from build123d import *

# Parameters (mm, degrees)
SKETCH1_R                = 50
BOSS_EXTRUDE1_DEPTH      = 50
BOSS_EXTRUDE2_REACH      = 251.325
BOSS_EXTRUDE2_END_RADIUS = 65
BOSS_EXTRUDE2_START      = 120
SKETCH2_R                = 45
SKETCH4_R                = 5
CUT_EXTRUDE1_DEPTH       = 20
FILLET1_R                = 5
FILLET2_R                = 1
FILLET3_R                = 3


with BuildPart() as part:
    # Sketch1 → Boss-Extrude1 (new, symmetric)
    with BuildSketch(Plane.XY):
        with BuildLine():
            Line((-100, -40), (-100, 40))
            Line((-100, 40), (-17.173936855, 62.690157863))
            ThreePointArc((-17.173936855, 62.690157863), (65, 0), (-17.173936855, -62.690157863))
            Line((-17.173936855, -62.690157863), (-100, -40))
        make_face()
        Circle(SKETCH1_R, mode=Mode.SUBTRACT)
    extrude(amount=BOSS_EXTRUDE1_DEPTH, both=True)

    # Boss-Extrude2: up to this cylinder (the profile starts outside it)
    boss_extrude2_end = Plane(origin=(0, 0, 0), z_dir=(0, 0, -1)) * Cylinder(BOSS_EXTRUDE2_END_RADIUS, 633.65, mode=Mode.PRIVATE)
    # Sketch2 → Boss-Extrude2 (add, up to the surface)
    with BuildSketch(Plane(origin=(0, 0, 0), x_dir=(0, 0, -1), z_dir=(1, 0, 0)).offset(BOSS_EXTRUDE2_START), mode=Mode.PRIVATE) as boss_extrude2_sk1:
        Circle(SKETCH2_R)
    boss_extrude2_tool1 = extrude(boss_extrude2_sk1.sketch, amount=-BOSS_EXTRUDE2_REACH, mode=Mode.PRIVATE) - boss_extrude2_end
    add(boss_extrude2_tool1.solids().sort_by_distance((120, 0, 0))[0])

    # Sketch3 → Revolve1 (revolve)
    with BuildSketch(Plane.XY):
        Polygon((120, 0), (180, 0), (172.019237886, -4.607695155), (164.019237886, -4.607695155), (164.019237886, -9.226497308), (154.019237886, -15), (154.019237886, -25), (139.019237886, -25), (139.019237886, -20), (120, -20), align=None)
    revolve(axis=Axis((0, 0, 0), (1, 0, 0)))

    # Sketch4 → Cut-Extrude1 (cut)
    with BuildSketch(Plane(origin=(120, 0, 0), x_dir=(0, 0, -1), z_dir=(1, 0, 0))):
        with Locations((0, 35)):
            Circle(SKETCH4_R)
        with Locations((35, 0)):
            Circle(SKETCH4_R)
        with Locations((0, -35)):
            Circle(SKETCH4_R)
        with Locations((-35, 0)):
            Circle(SKETCH4_R)
    extrude(amount=-CUT_EXTRUDE1_DEPTH, mode=Mode.SUBTRACT)

    # Fillet1
    fillet1_edges = [part.edges().sort_by_distance(p)[0] for p in [
        (120, 20, 0),
        (139.019237886, 20, 0),
    ]]
    fillet(fillet1_edges, radius=FILLET1_R - 0.0001)  # a hair under: the kernel refuses the full size

    # Fillet2
    fillet2_edges = [part.edges().sort_by_distance(p)[0] for p in [
        (-58.586968427, 51.345078932, 50),
        (-58.586968427, -51.345078932, 50),
        (-58.586968427, 51.345078932, -50),
        (65, 0, -50),
        (-58.586968427, -51.345078932, -50),
        (65, 0, 50),
    ]]
    fillet(fillet2_edges, radius=FILLET2_R)

    # Fillet3
    fillet3_edges = [part.edges().sort_by_distance(p)[0] for p in [
        (154.019237886, 25, 0),
        (139.019237886, 25, 0),
    ]]
    fillet(fillet3_edges, radius=FILLET3_R)


solid = part.part
CAD build for the part. Positions are in the model's coordinates, mm. A direction names the side the tool comes from. Round coordinates to 2 decimals unless told otherwise and drop trailing zeros. Loops run counter-clockwise (first coordinate to the right, second up) from the corner with the lowest first, then second, coordinate; pieces in that order, holes last. Notation, with made-up numbers: M 2.5,36 L 47.5,36 A13 cw 47.5,44 Z; hole C -19.5,1.5 d2. An arc over 180 degrees is marked long. One line per question, with ' | ' between items. Start each with the question number.
Item 1: Cut at B-B, the plane x = 148. Write the cut outline in (y, z).
Item 2: Two-plate mould, pull along Z, no slides. Class faces 4 (the cylindrical face through (110, 39, -3)), 5 (the flat face through (-53, 1, -50)), 6 (the flat face through (-58.007, -51.504, 0.686)): pulls with the +Z half, pulls with the -Z half, needs draft (parallel to the pull), parting line crosses it, or undercut.
Item 3: Cut at A-A, the plane z = 35. Write the cut outline in (x, y).
Item 4: Which spindle directions (+Z, -Z, +X, -X, +Y, -Y) get a long thin tool onto all of the face, cutting with end or side? Do faces 1 (the cylindrical face through (146.16, -23.846, -7.509)), 2 (the flat face through (-59.167, 51.186, 0.686)), 3 (the cylindrical face through (129.446, 4.336, 19.524)). Say none if no direction does.
Item 5: Pin check, flat tips, straight feed: pin 1 Ø13 at (y, z) = (0, 35) entering from +X; pin 2 Ø6 at (y, z) = (0.5, -19.5) entering from +X; pin 3 Ø1.5 at (x, z) = (-7, -16) entering from +Y. Stop position of each tip, or through.
Item 6: Wall check: line 1 (Y direction, x = 115, z = 0); line 2 (X direction, y = 10, z = -10); line 3 (X direction, y = 36, z = -37). Give the ranges that are in metal, low to high.
Responses:
1) outline: C 0,0 d50
2) face 4: undercut | face 5: pulls with the -Z half | face 6: needs draft
3) outline: M -100,-40 L -17.17,-62.69 A65 ccw 58.52,-28.28 L 120,-28.28 L 120,-5 L 100,-5 L 100,5 L 120,5 L 120,28.28 L 58.52,28.28 A65 ccw -17.17,62.69 L -100,40 Z; hole C 0,0 d100
4) face 1: +X | face 2: +Z, -Z, -X, +Y | face 3: none
5) pin 1: stops at x = 120 | pin 2: stops at x = 154.02 | pin 3: stops at y = 64.7
6) line 1: y = -45 to -40, -30 to 30, 40 to 45 | line 2: x = -100 to -48.99, 48.99 to 155.51 | line 3: x = -100 to -34.7, 34.7 to 54.12
